from build123d import *

# Parameters (mm, degrees)
SKETCH_1_W           = 40
SKETCH_1_H           = 60
SKETCH_1_R           = 3.05
EXTRUDE_1_DEPTH      = 3
SKETCH_2_W           = 40
SKETCH_2_H           = 4
EXTRUDE_2_DEPTH      = 45
EXTRUDE_3_DEPTH      = 20
EXTRUDE_3_DEPTH_BACK = 20
SKETCH_4_W           = 10
SKETCH_4_H           = 15.081171456
SKETCH_4_R           = 3.05
SKETCH_4_H_2         = 5
SKETCH_4_H_3         = 20.081171456
CUT_EXTRUDE_1_DEPTH  = 58.662812973


with BuildPart() as part:
    # Sketch 1 → Extrude 1 (new body)
    with BuildSketch(Plane(origin=(0, 0, 0), x_dir=(1, 0, 0), z_dir=(0, 1, 0))):
        Rectangle(SKETCH_1_W, SKETCH_1_H)
        with Locations(Location((-12.5, 12.5, 0), (0, 0, 270))):
            Circle(SKETCH_1_R, mode=Mode.SUBTRACT)
        with Locations(Location((12.5, 12.5, 0), (0, 0, 90))):
            Circle(SKETCH_1_R, mode=Mode.SUBTRACT)
        with Locations(Location((12.5, -12.5, 0), (0, 0, 270))):
            Circle(SKETCH_1_R, mode=Mode.SUBTRACT)
        with Locations(Location((-12.5, -12.5, 0), (0, 0, 90))):
            Circle(SKETCH_1_R, mode=Mode.SUBTRACT)
    extrude(amount=EXTRUDE_1_DEPTH)

    # Sketch 2 → Extrude 2 (add)
    with BuildSketch(Plane(origin=(0, 3, 0), x_dir=(1, 0, 0), z_dir=(0, 1, 0))):
        with Locations((0, 3)):
            Rectangle(SKETCH_2_W, SKETCH_2_H)
        with Locations((0, -3)):
            Rectangle(SKETCH_2_W, SKETCH_2_H)
    extrude(amount=EXTRUDE_2_DEPTH)

    # Sketch 3 → Extrude 3 (add, two sides: drawn at the far end of the back side and taken through both)
    with BuildSketch(Plane(origin=(0, 0, 0), x_dir=(0, 0, -1), z_dir=(1, 0, 0)).offset(-EXTRUDE_3_DEPTH_BACK)):
        Polygon((-5, 29.121355199), (-20.081171456, 3), (-25.081171456, 3), (-5, 37.781609237), align=None)
        Polygon((5, 37.781609237), (5, 29.121355199), (20.081171456, 3), (25.081171456, 3), align=None)
    extrude(amount=EXTRUDE_3_DEPTH + EXTRUDE_3_DEPTH_BACK)

    # Sketch 4 → Cut-Extrude 1 (cut, through all)
    # profile 1 of 8: a face of its own
    with BuildSketch(Plane(origin=(0, 3, 0), x_dir=(1, 0, 0), z_dir=(0, 1, 0))):
        with Locations((12.5, -12.540585728)):
            Rectangle(SKETCH_4_W, SKETCH_4_H)
        with Locations(Location((12.5, -12.5, 0), (0, 0, 270))):
            Circle(SKETCH_4_R, mode=Mode.SUBTRACT)
    # profile 2 of 8: a face of its own
    with BuildSketch(Plane(origin=(0, 3, 0), x_dir=(1, 0, 0), z_dir=(0, 1, 0))):
        with Locations(Location((12.5, -12.5, 0), (0, 0, 270))):
            Circle(SKETCH_4_R)
    # profile 3 of 8: a face of its own
    with BuildSketch(Plane(origin=(0, 3, 0), x_dir=(1, 0, 0), z_dir=(0, 1, 0))):
        with Locations((12.5, -22.581171456)):
            Rectangle(SKETCH_4_W, SKETCH_4_H_2)
    # profile 4 of 8: a face of its own
    with BuildSketch(Plane(origin=(0, 3, 0), x_dir=(1, 0, 0), z_dir=(0, 1, 0))):
        with Locations((-12.5, -12.540585728)):
            Rectangle(SKETCH_4_W, SKETCH_4_H)
        with Locations(Location((-12.5, -12.5, 0), (0, 0, 90))):
            Circle(SKETCH_4_R, mode=Mode.SUBTRACT)
    # profile 5 of 8: a face of its own
    with BuildSketch(Plane(origin=(0, 3, 0), x_dir=(1, 0, 0), z_dir=(0, 1, 0))):
        with Locations(Location((-12.5, -12.5, 0), (0, 0, 90))):
            Circle(SKETCH_4_R)
    # profile 6 of 8: a face of its own
    with BuildSketch(Plane(origin=(0, 3, 0), x_dir=(1, 0, 0), z_dir=(0, 1, 0))):
        with Locations((-12.5, -22.581171456)):
            Rectangle(SKETCH_4_W, SKETCH_4_H_2)
    # profile 7 of 8: a face of its own
    with BuildSketch(Plane(origin=(0, 3, 0), x_dir=(1, 0, 0), z_dir=(0, 1, 0))):
        with Locations((-12.5, 15.040585728)):
            Rectangle(SKETCH_4_W, SKETCH_4_H_3)
    # profile 8 of 8: a face of its own
    with BuildSketch(Plane(origin=(0, 3, 0), x_dir=(1, 0, 0), z_dir=(0, 1, 0))):
        with Locations((12.5, 15.040585728)):
            Rectangle(SKETCH_4_W, SKETCH_4_H_3)
    extrude(amount=CUT_EXTRUDE_1_DEPTH, mode=Mode.SUBTRACT)


solid = part.part
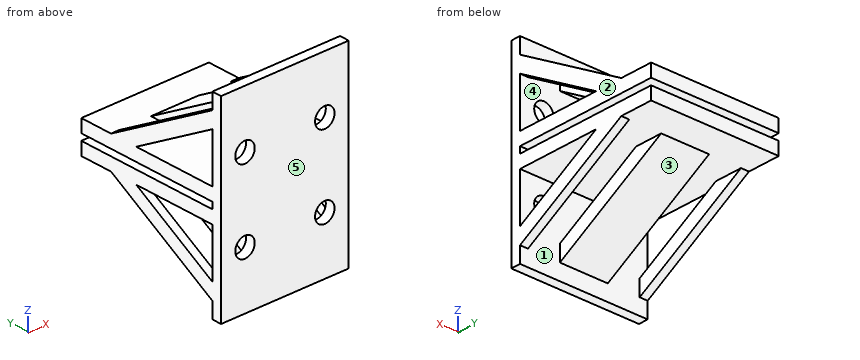
Read the model definition and answer for the solid it produces. Units are mm, in the model's axes. Face numbers are marked on the shaded views. A direction names the side the tool comes from. Give positions to 0.01 mm unless a question says otherwise; leave off trailing zeros. Write each loop counter-clockwise with the first axis right and the second up, starting at its lowest first coordinate (ties: lowest second). Pieces come first, ordered by that corner, then holes. Notation, with made-up numbers: (13.5, 24) - (26.5, 24) arc R31 cw to (26.5, 56) - close; hole circle Ø6 at (16, 65). An arc over 180 degrees is marked (long way). Answer in a Markdown table with one row per item. Add a question column.
Item 1: Section C-C, the plane z = 13.5 is taken. Write down the section's boundary in (x, y).
Item 2: A tool of negligible diameter and unlimited length cuts with its end or side. For the marked faces 4 and 5, from which of +Z, -Z, +X, -X, +Y, -Y can it reach the whole face along a straight path? Write none if from no direction.
Item 3: Find the intervals of material crossed by L1, parallel to X at y = 1.7, z = -12.5; L2, parallel to Z at x = 16.5, y = 29; L3, parallel to X at y = 19, z = -13, in increasing order.
Item 4: Section D-D, the plane y = 11 is taken. Count the separate pieces of the cut face and the enclosed holes in it, and give its area (3 significant figures).
Item 5: Section A-A, the plane x = 12.5 is taken. Write down the section's boundary in (y, z).
Item 6: Flat-ended cylindrical pins translate along their axes: P1, Ø10, axis at x = 10.5, y = 15.5, coming from the +Z side; P2, Ø1, axis at x = -16, y = 25.5, coming from the -Z side; P3, Ø10, axis at y = 27, z = -13, coming from the +X side; P4, Ø1.6, axis at x = 4.5, z = 0, coming from the +Y side. Find the tip coordinate at first contact, or state that the pin passes through.
Item 7: Determine the mould class of the marked faces 1, 2 and 3 for opening direction Z: pulls with the +Z half, pulls with the -Z half, needs draft (parallel to the pull), parting line crosses it, or undercut.
Item 8: Section B-B, the plane y = 41 is taken. Write down the section's boundary in (x, z), and give its area (3 significant figures).
Recorded:
| question | item | result |
|---|---|---|
| 1 | outline | (-20, 0) - (-15.38, 0) - (-15.38, 3) - (-20, 3) - close; (-20, 14.4) - (-17.5, 14.4) - (-17.5, 23.06) - (-20, 23.06) - close; (-9.62, 0) - (9.62, 0) - (9.62, 3) - (-9.62, 3) - close; (-7.5, 14.4) - (7.5, 14.4) - (7.5, 23.06) - (-7.5, 23.06) - close; (15.38, 0) - (20, 0) - (20, 3) - (15.38, 3) - close; (17.5, 14.4) - (20, 14.4) - (20, 23.06) - (17.5, 23.06) - close |
| 2 | face 4 | none |
| 2 | face 5 | +Z, -Z, +X, -X, -Y |
| 3 | L1 | x = -20 to -15.55, -9.45 to 9.45, 15.55 to 20 |
| 3 | L2 | z = -5 to -1, 1 to 5 |
| 3 | L3 | x = -20 to -17.5, -7.5 to 7.5, 17.5 to 20 |
| 4 | separate pieces | 8 |
| 4 | enclosed holes | 0 |
| 4 | area | 520 mm2 |
| 5 | outline | (0, -30) - (3, -30) - (3, -15.55) - (0, -15.55) - close; (0, -9.45) - (3, -9.45) - (3, -5) - (48, -5) - (48, -1) - (3, -1) - (3, 1) - (48, 1) - (48, 5) - (3, 5) - (3, 9.45) - (0, 9.45) - close; (0, 15.55) - (3, 15.55) - (3, 30) - (0, 30) - close |
| 6 | P1 | stops at z = 20.17 |
| 6 | P2 | stops at z = -5 |
| 6 | P3 | stops at x = 20 |
| 6 | P4 | stops at y = 3 |
| 7 | face 1 | undercut |
| 7 | face 2 | needs draft |
| 7 | face 3 | pulls with the -Z half |
| 8 | outline | (-20, -5) - (20, -5) - (20, -1) - (-20, -1) - close; (-20, 1) - (20, 1) - (20, 5) - (-20, 5) - close |
| 8 | area | 320 mm2 |
